Can you work these out from the model? Positions are in its coordinate system, mm. Face numbers are marked on the shaded views. A direction names the side the tool comes from. Coordinates: 2 decimals unless noted, no trailing zeros. Order: outer loops, then holes, each group sorted by start corner. A loop starts at its lowest first (then second) coordinate and runs counter-clockwise, first axis right, second up. Notation, with made-up numbers: M 43,48.5 L 80,48.5 A20 cw 80,64.5 Z; hole C 72,-25 d1. An arc over 180 degrees is marked long. Answer as a JSON object with one key per item and string values.
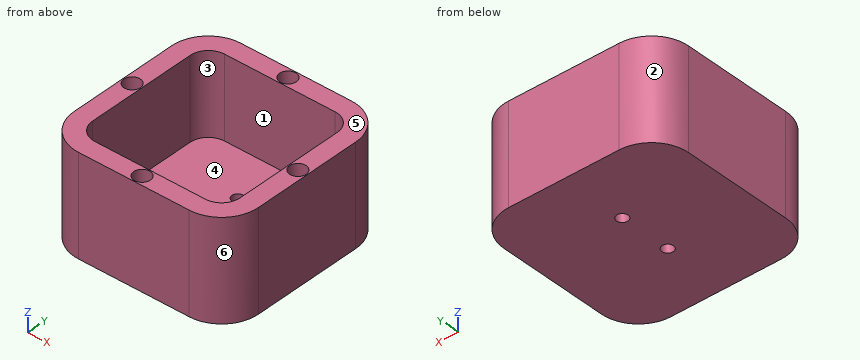
from build123d import *

# Parameters (mm, degrees)
SKETCH1_W           = 50
SKETCH1_H           = 50
BOSS_EXTRUDE1_DEPTH = 27
FILLET1_R           = 10
SHELL1_T            = -5
SKETCH3_R           = 1.55
CUT_EXTRUDE1_DEPTH  = 5
SKETCH4_R           = 2.25
CUT_EXTRUDE2_DEPTH  = 5


with BuildPart() as part:
    # Sketch1 → Boss-Extrude1 (new body)
    with BuildSketch(Plane.XY):
        with Locations((25, 25)):
            Rectangle(SKETCH1_W, SKETCH1_H)
    extrude(amount=BOSS_EXTRUDE1_DEPTH)

    # Fillet1
    fillet1_edges = [part.edges().sort_by_distance(p)[0] for p in [
        (0, 50, 13.5),
        (50, 50, 13.5),
        (50, 0, 13.5),
        (0, 0, 13.5),
    ]]
    fillet(fillet1_edges, radius=FILLET1_R)

    # Shell1
    shell1_openings = [part.faces().sort_by_distance(p)[0] for p in [
        (25, 25, 27),
    ]]
    offset(amount=SHELL1_T, openings=shell1_openings, kind=Kind.INTERSECTION)

    # Sketch3 → Cut-Extrude1 (cut)
    with BuildSketch(Plane.XY.offset(5)):
        with Locations((25, 32)):
            Circle(SKETCH3_R)
        with Locations((25, 18)):
            Circle(SKETCH3_R)
    extrude(amount=-CUT_EXTRUDE1_DEPTH, mode=Mode.SUBTRACT)

    # Sketch4 → Cut-Extrude2 (cut)
    with BuildSketch(Plane.XY.offset(27)):
        with Locations((25, 2.5)):
            Circle(SKETCH4_R)
        with Locations((2.5, 25)):
            Circle(SKETCH4_R)
        with Locations((25, 47.5)):
            Circle(SKETCH4_R)
        with Locations((47.5, 25)):
            Circle(SKETCH4_R)
    extrude(amount=-CUT_EXTRUDE2_DEPTH, mode=Mode.SUBTRACT)


solid = part.part
Item 1: I want a section at C-C, the plane y = 32. Write out the boundary of the cut face in (x, z), plus the area to 4 significant figures.
Answers follow:
{"outline": "M 0,0 L 23.45,0 L 23.45,5 L 5,5 L 5,27 L 0,27 Z; M 26.55,0 L 50,0 L 50,27 L 45,27 L 45,5 L 26.55,5 Z", "area": "454.5 mm^2"}
Item 2: I want a section at D-D, the plane z = 3.5. Write out the boundary of the cut face in (x, y), plus the area to 3 significant figures.
Answers follow:
{"outline": "M 0,10 A10 ccw 10,0 L 40,0 A10 ccw 50,10 L 50,40 A10 ccw 40,50 L 10,50 A10 ccw 0,40 Z; hole C 25,18 d3.1; hole C 25,32 d3.1", "area": "2,400 mm^2"}
Item 3: Please list where these lines run through material, in increasing order: line 1 (Y direction, x = 25, z = 23.15); line 2 (Y direction, x = 25, z = 3.55); line 3 (X direction, y = 32.5, z = 13.5).
Answers follow:
{"line 1": "y = 0 to 0.25, 4.75 to 5, 45 to 45.25, 49.75 to 50", "line 2": "y = 0 to 16.45, 19.55 to 30.45, 33.55 to 50", "line 3": "x = 0 to 5, 45 to 50"}
Item 4: I'm going to push flat-ended pins straight in: pin 1 (1.5 mm diameter, centred on x = 9.5, z = 18.5, fed in from +Y); pin 2 (4 mm diameter, centred on x = 25, y = 32, fed in from +Z); pin 3 (2 mm diameter, centred on x = 47, y = 24, fed in from +Z). Where does each tip first touch, or does it pass through?
Answers follow:
{"pin 1": "stops at y = 50", "pin 2": "stops at z = 5", "pin 3": "stops at z = 22"}
Item 5: I want a section at B-B, the plane z = 25.5. Write out the boundary of the cut face in (x, y).
Answers follow:
{"outline": "M 0,10 A10 ccw 10,0 L 40,0 A10 ccw 50,10 L 50,40 A10 ccw 40,50 L 10,50 A10 ccw 0,40 Z; hole C 2.5,25 d4.5; hole M 5,10 A5 ccw 10,5 L 40,5 A5 ccw 45,10 L 45,40 A5 ccw 40,45 L 10,45 A5 ccw 5,40 Z; hole C 25,2.5 d4.5; hole C 25,47.5 d4.5; hole C 47.5,25 d4.5"}
Item 6: If we mould it in two halves opening along X, with no side actions, what happens to the marked faces 3, 4, 5 and 6? For each: pulls with the +X half, pulls with the -X half, needs draft (parallel to the pull), parting line crosses it, or undercut.
Answers follow:
{"face 3": "undercut", "face 4": "undercut", "face 5": "needs draft", "face 6": "pulls with the +X half"}
Item 7: Which directions (+Z, -Z, +X, -X, +Y, -Y) give clear straight access to the entire face, cutting with the end or side of a thin tool? Please do the marked faces 1 and 2.
Answers follow:
{"face 1": "+Z", "face 2": "+Z, -Z, -X, +Y"}
Item 8: I want a section at A-A, the plane x = 25. Write out the boundary of the cut face in (y, z), plus the area to 3 significant figures.
Answers follow:
{"outline": "M 0,0 L 16.45,0 L 16.45,5 L 5,5 L 5,27 L 4.75,27 L 4.75,22 L 0.25,22 L 0.25,27 L 0,27 Z; M 19.55,0 L 30.45,0 L 30.45,5 L 19.55,5 Z; M 33.55,0 L 50,0 L 50,27 L 49.75,27 L 49.75,22 L 45.25,22 L 45.25,27 L 45,27 L 45,5 L 33.55,5 Z", "area": "394 mm^2"}
